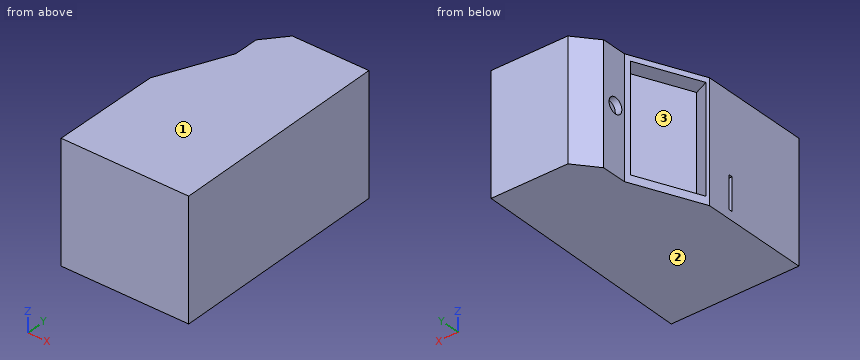
```python
from build123d import *

# Parameters (mm, degrees)
PAD_DEPTH       = 90
SKETCH001_W     = 49.773563
SKETCH001_H     = 80.123774
POCKET_DEPTH    = 12
SKETCH002_R     = 5.887963
POCKET001_DEPTH = 5
SKETCH003_W     = 2.713595
SKETCH003_H     = 24.526356
POCKET002_DEPTH = 5


with BuildPart() as part:
    # Sketch → Pad (new body)
    with BuildSketch(Plane.XY):
        Polygon((-48.492157, 7.780759), (-47.988304, -74.853439), (48.754147, -74.349571), (45.227108, 95.453613), (-12.717616, 94.949745), (-26.322012, 78.322136), (-26.322012, 59.175186), align=None)
    extrude(amount=PAD_DEPTH)

    # Sketch001 (on Face7 of Pad) → Pocket (cut)
    with BuildSketch(Plane(origin=(-43.714137, 18.857079, 0), x_dir=(-0.396091, -0.918211, 0), z_dir=(-0.918211, 0.396091, 0))):
        with Locations((-15.26545, 45.985601)):
            Rectangle(SKETCH001_W, SKETCH001_H)
    extrude(amount=-POCKET_DEPTH, mode=Mode.SUBTRACT)

    # Sketch002 (on Face6 of Pocket) → Pocket001 (cut)
    with BuildSketch(Plane(origin=(-26.322012, 0, 0), x_dir=(0, -1, 0), z_dir=(-1, 0, 0))):
        with Locations((-67.568731, 49.26139)):
            Circle(SKETCH002_R)
    extrude(amount=-POCKET001_DEPTH, mode=Mode.SUBTRACT)

    # Sketch003 (on Face1 of Pocket001) → Pocket002 (cut)
    with BuildSketch(Plane(origin=(-48.442914, -0.295375, 0), x_dir=(0.006097, -0.999981, 0), z_dir=(-0.999981, -0.006097, 0))):
        with Locations((11.426969, 18.839719)):
            Rectangle(SKETCH003_W, SKETCH003_H)
    extrude(amount=-POCKET002_DEPTH, mode=Mode.SUBTRACT)


solid = part.part
```
Here's how the part is built. I have some questions about the finished solid (model axes, mm). Face numbers are marked on the shaded views. Give positions to 0.01 mm unless a question says otherwise; leave off trailing zeros. Write each loop counter-clockwise with the first axis right and the second up, starting at its lowest first coordinate (ties: lowest second). Pieces come first, ordered by that corner, then holes.
(1) Imagine slicing it at A-A, the plane z = 36.5. Write out the boundary of the cut face in (x, y), and give its area (3 significant figures).
Output values:
outline: (-48.49, 7.78) - (-47.99, -74.85) - (48.75, -74.35) - (45.23, 95.45) - (-12.72, 94.95) - (-26.32, 78.32) - (-26.32, 59.18) - (-27.81, 55.73) - (-16.79, 50.97) - (-36.51, 5.27) - (-47.53, 10.02) - close
area: 14,100 mm2
(2) Imagine slicing it at D-D, the plane z = 21. Write out the boundary of the cut face in (x, y).
Output values:
outline: (-48.49, 7.78) - (-48.38, -10.37) - (-43.38, -10.33) - (-43.37, -13.05) - (-48.36, -13.08) - (-47.99, -74.85) - (48.75, -74.35) - (45.23, 95.45) - (-12.72, 94.95) - (-26.32, 78.32) - (-26.32, 59.18) - (-27.81, 55.73) - (-16.79, 50.97) - (-36.51, 5.27) - (-47.53, 10.02) - close
(3) Thinking about a two-plate mould opening in Z: for the marked faces 1, 2 and 3, which applies, pulls with the +Z half, pulls with the -Z half, needs draft (parallel to the pull), parting line crosses it, or undercut?
Output values:
face 1: pulls with the +Z half
face 2: pulls with the -Z half
face 3: undercut
(4) Imagine slicing it at C-C, the plane x = -32. Write out the boundary of the cut face in (y, z), and give its area (3 significant figures).
Output values:
outline: (-74.77, 0) - (46.01, 0) - (46.01, 5.92) - (15.72, 5.92) - (15.72, 86.05) - (46.01, 86.05) - (46.01, 90) - (-74.77, 90) - close
area: 8,440 mm2
(5) Will these pins go through, and if not, where does the flat tip stop? pin 1 (9.5 mm diameter, centred on y = 64.5, z = 33, fed in from -X); pin 2 (5 mm diameter, centred on y = -2, z = 28, fed in from -X); pin 3 (1 mm diameter, centred on y = 6, z = 63.5, fed in from +X).
Output values:
pin 1: stops at x = -26.32
pin 2: stops at x = -48.45
pin 3: stops at x = 47.1
(6) Imagine slicing it at B-B, the plane y = 43. Write out the boundary of the cut face in (x, z), and give its area (3 significant figures).
Output values:
outline: (-33.3, 0) - (46.32, 0) - (46.32, 90) - (-33.3, 90) - (-33.3, 86.05) - (-20.23, 86.05) - (-20.23, 5.92) - (-33.3, 5.92) - close
area: 6,120 mm2
(7) If I drill on L1, parallel to Y at x = 36.5, z = 81; L2, parallel to X at y = 45.5, z = 54.5; L3, parallel to X at y = 53.5, z = 55.5, over which ranges is the centre line in solid material (lowest first)?
Output values:
L1: y = -74.41 to 95.38
L2: x = -19.15 to 46.26
L3: x = -22.65 to 46.1
